from build123d import *

# Parameters (mm, degrees)
F0_W     = 12
F0_H     = 40
F1_DEPTH = 4
F2_W     = 5
F2_H     = 40
F3_DEPTH = 2
F4_R     = 1.5
F5_DEPTH = 25
F6_R     = 1.5
F7_DEPTH = 2
F8_W     = 4.029665
F8_H     = 26
F8_W_2   = 12
F9_DEPTH = 25


with BuildPart() as f1:
    # F0 (on Front) → F1 (new body)
    with BuildSketch(Plane.XZ):
        Rectangle(F0_W, F0_H)
    extrude(amount=F1_DEPTH)

    # F2 (on face) → F3 (join)
    with BuildSketch(Plane.XZ.offset(4)):
        Rectangle(F2_W, F2_H)
    extrude(amount=F3_DEPTH)

    # F4 (on face) → F5 (cut)
    with BuildSketch(Plane.XZ.offset(6)):
        with Locations((0, 16.5)):
            Circle(F4_R)
        with Locations((0, -13.5)):
            Circle(F4_R)
    extrude(amount=-F5_DEPTH, mode=Mode.SUBTRACT)

    # F6 (on face) → F7 (cut)
    with BuildSketch(Plane(origin=(0, 0, 0), x_dir=(-1, 0, 0), z_dir=(0, 1, 0))):
        Polygon((2.75, 14.912287), (2.75, 18.087713), (0, 19.675426), (-2.75, 18.087713), (-2.75, 14.912287), (0, 13.324574), align=None)
        with Locations((0, 16.5)):
            Circle(F6_R, mode=Mode.SUBTRACT)
        Polygon((2.750551, -11.913241), (0.001102, -10.324574), (-2.749449, -11.911332), (-2.750551, -15.086759), (-0.001102, -16.675426), (2.749449, -15.088668), align=None)
        with Locations((0, -13.5)):
            Circle(F6_R, mode=Mode.SUBTRACT)
    extrude(amount=-F7_DEPTH, mode=Mode.SUBTRACT)

    # F8 (on face) → F9 (cut)
    with BuildSketch(Plane(origin=(0, 0, 0), x_dir=(-1, 0, 0), z_dir=(0, 1, 0))):
        with Locations((8.014833, 7)):
            Rectangle(F8_W, F8_H)
        with Locations((0, 7)):
            Rectangle(F8_W_2, F8_H)
        Polygon((2.75, 18.087713), (2.75, 14.912287), (0, 13.324574), (-2.75, 14.912287), (-2.75, 18.087713), (0, 19.675426), align=None, mode=Mode.SUBTRACT)
        Polygon((0, 13.324574), (2.75, 14.912287), (2.75, 18.087713), (0, 19.675426), (-2.75, 18.087713), (-2.75, 14.912287), align=None)
    extrude(amount=-F9_DEPTH, mode=Mode.SUBTRACT)


solid = f1.part
Design review of the part built by this model. Coordinates are the model's own, in mm. A direction names the side the tool comes from. Round coordinates to 2 decimals unless told otherwise and drop trailing zeros. Write each loop counter-clockwise with the first axis right and the second up, starting at its lowest first coordinate (ties: lowest second). Pieces come first, ordered by that corner, then holes. Notation, with made-up numbers: (9, -34) - (41, -34) arc R18 cw to (41, -14) - close; hole circle Ø11 at (16.25, -31.5). An arc over 180 degrees is marked (long way). Return JSON: item names as keys, results as strings. Group by question number.
Item 1: We need section B-B on z = -13.5. Write out the cut boundary in (x, y), and give its area (3 significant figures).
Item 2: The part is to be moulded in two halves that separate along X. For faces 4 (the face through (4, -4, -13)), 5 (the face through (2.5, -5, -13)), 6 (the face through (1.355, -0.986, -11.107)), 7 (the face through (0, -4, -15)), say which applies: pulls with the +X half, pulls with the -X half, needs draft (parallel to the pull), parting line crosses it, or undercut.
Item 3: We need section D-D on x = -0.5. Write out the cut boundary in (y, z).
Item 4: For probe 1 along Z at (x, y) = (0, -4.4); probe 2 along X at (y, z) = (-5.05, -13.5); probe 3 along X at (y, z) = (-2.85, -13.5), list the stretches that pass through material, from the lowest coordinate up. Write a range as [from, to].
Item 5: We need section A-A on y = -1.6. Write out the cut boundary in (x, z).
Item 6: We need section C-C on z = -8.75. Write out the cut boundary in (x, y), and give its area (3 significant figures).
Item 7: Machinability: for faces 1 (the face through (-2.5, -5, -13)), 2 (the face through (1, -2, -15)), 3 (the face through (-3, 0, -13)), which of the approach directions +Z, -Z, +X, -X, +Y, -Y give a long, thin tool a straight path to every point of the face, cutting with its end or side? Answer none if there is none.
Item 8: Insertion check: P1, Ø4, axis at x = 5, z = -12, coming from the -Y side; P2, Ø1.6, axis at y = -5.5, z = -11.5, coming from the +X side; P3, Ø1, axis at y = -5, z = -11, coming from the -X side; P4, Ø1, axis at x = 3.5, y = -5.5, coming from the -Z side. Each pin has a flat end and moves straight along its axis. Give the tip position at first contact, or say it passes through.
Model answer:
{
 "1": {"outline": "(-6, -4) - (-2.5, -4) - (-2.5, -6) - (-1.5, -6) - (-1.5, -2) - (-2.75, -2) - (-2.75, 0) - (-6, 0) - close; (1.5, -6) - (2.5, -6) - (2.5, -4) - (6, -4) - (6, 0) - (2.75, 0) - (2.75, -2) - (1.5, -2) - close", "area": "35.0 mm²"},
 "2": {"face 4": "needs draft", "face 5": "pulls with the +X half", "face 6": "undercut", "face 7": "undercut"},
 "3": {"outline": "(-6, -20) - (0, -20) - (0, -16.39) - (-2, -16.39) - (-2, -14.91) - (-6, -14.91) - close; (-6, -12.09) - (-2, -12.09) - (-2, -10.61) - (0, -10.61) - (0, -6) - (-6, -6) - close"},
 "4": {"probe 1": "z = [-20, -15], [-12, -6]", "probe 2": "x = [-2.5, -1.5], [1.5, 2.5]", "probe 3": "x = [-6, -1.5], [1.5, 6]"},
 "5": {"outline": "(-6, -20) - (6, -20) - (6, -6) - (-6, -6) - close; hole (-2.75, -15.09) - (0, -16.68) - (2.75, -15.09) - (2.75, -11.91) - (0, -10.32) - (-2.75, -11.91) - close"},
 "6": {"outline": "(-6, -4) - (-2.5, -4) - (-2.5, -6) - (2.5, -6) - (2.5, -4) - (6, -4) - (6, 0) - (-6, 0) - close", "area": "58.0 mm²"},
 "7": {"face 1": "+Z, -Z, -X, -Y", "face 2": "+Y", "face 3": "+Z, -Z, +X, -X, +Y"},
 "8": {"P1": "stops at y = -4", "P2": "stops at x = 2.5", "P3": "stops at x = -2.5", "P4": "passes through"}
}
